The listing builds one solid part. Answer for the finished solid, in the listing's coordinates (mm). A direction names the side the tool comes from. Round coordinates to 2 decimals unless told otherwise and drop trailing zeros. Loops run counter-clockwise (first coordinate to the right, second up) from the corner with the lowest first, then second, coordinate; pieces in that order, holes last. Notation, with made-up numbers: (-35, 28) -> (-19, 28) arc R9 ccw to (-19, 35) -> close; hole circle Ø3 at (-25, 18). An arc over 180 degrees is marked (long way). Write each question's results on one line, items separated by ' | '. Start each with the question number.
(1) Flat-ended cylindrical pins translate along their axes: pin 1 (4 mm diameter, centred on y = -11.5, z = -11.5, fed in from +X); pin 2 (3 mm diameter, centred on x = 25.5, z = -13.5, fed in from +Y) (3 decimals); pin 3 (3.5 mm diameter, centred on x = 39.5, z = 0, fed in from +Y); pin 4 (2.5 mm diameter, centred on x = 5.5, y = -19.875, fed in from +Z). Find the tip coordinate at first contact, or state that the pin passes through.
(2) Straight lines are drawn through the part: probe 1 along Y at (x, z) = (5.5, -2.75) (3 decimals); probe 2 along Y at (x, z) = (39.5, 0.3); probe 3 along X at (y, z) = (-16.75, -3). For each, find the intervals that lie inside material, in ascending order.
(3) The part is cut by section B-B (z = 1). Determine the outline of the cut face in (x, y) (3 decimals).
(4) The part is cut by section D-D (y = -19.25). Determine the outline of the cut face in (x, z), plus the area to 3 significant figures.
(5) Determine the mould class of faces 4 (the face through (25, -11, 13.25)), 5 (the face through (25, -12.975, -14)), 6 (the face through (37, -11, -2)), 7 (the face through (24.73, -10.45, 15.78)) for opening direction Y: released by +Y, released by -Y, zero draft, split by the parting line, or undercut.
(6) The part is cut by section A-A (x = 5.5). Determine the outline of the cut face in (y, z) (3 decimals).
(7) The part is cut by section C-C (x = 25.47). Determine the outline of the cut face in (y, z) (3 decimals).
(8) For faces 1 (the face through (13, -9.8, -10.2)), 2 (the face through (14.24, -13.11, 10.24)), 3 (the face through (14, -11, -11.25)), determine the directions among +Z, -Z, +X, -X, +Y, -Y from which every point of the face is accessible in a straight line to the end or side of a thin tool.
Autodesk Inventor part; units mm, degrees
ref_plane "YZ Plane" through (0, 0, 0) normal (1, 0, 0) x (0, 1, 0)
ref_plane "XZ Plane" through (0, 0, 0) normal (0, 1, 0) x (-1, 0, 0)
ref_plane "XY Plane" through (0, 0, 0) normal (0, 0, 1) x (1, 0, 0)
sketch "Sketch1" plane through (0, 0, 0) normal (0, 0, 1) x (1, 0, 0)
  line L0 (0, 0) -> (32.875, 0)
  line L1 (37, 0) -> (37, -4.125)
  line L2 (37, -22.25) -> (0, -22.25)
  line L3 (0, -22.25) -> (0, -11.125)
  line L4 (0, -11.125) -> (37, -11.125) construction
  line L5 (0, -11.125) -> (0, 0)
  circle A0 centre (14.5, -11.125) radius 2
  circle A1 centre (5.5, -2.375) radius 1.5
  arc A2 (37, -4.125) -> (32.875, 0) centre (32.875, -4.125) ccw
  line L6 (32.875, 0) -> (37, 0)
  line L7 (37, -4.125) -> (37, -22.25)
  arc A3 (32.875, -22.25) -> (37, -18.125) centre (32.875, -18.125) ccw
  circle A4 centre (5.5, -19.875) radius 1.5
  circle A5 centre (25.47, -11.125) radius 2.7
  line L8 (23.5034, -9.275) -> (27.4366, -9.275)
  line L9 (27.4366, -12.975) -> (23.5034, -12.975)
  point P0 (36.5, -18.125)
  point P1 (36.9, -18.125)
  dimension "d6" = 4
  dimension "d8" = 3
  dimension "d11" = 5.5
  dimension "d12" = 22.25
  dimension "d13" = 8.75
  dimension "d16" = 14.5
  dimension "d17" = 14
  dimension "d18" = 37
  dimension "d19" = 3.7
  dimension "d28" = 5.4
  dimension "d29" = 11.53
extrude "Extrusion1" add sketch "Sketch1" along normal mid plane 18.5 contours L0 A2 L7 A3 L2 L3 L5
extrude "Extrusion2" add sketch "Sketch1" along normal mid plane 22.5 contours A0
extrude "Extrusion3" add sketch "Sketch1" along normal mid plane 20.5 contours A5 L9 L8 | L8 A5 | A5 L9
extrude "Extrusion4" add sketch "Sketch1" along normal mid plane 36.5 contours A5 L9 L8
sketch "Sketch2" plane through (0, -22.25, 9.25) normal (-1, 0, 0) x (0, 0, 1)
  point P0 (-9.25, 22.25)
sketch "Sketch3" plane through (0, 0, -18.25) normal (0, 0, -1) x (-1, 0, 0)
  circle A0 centre (-25.47, -11.125) radius 1
  arc A1 (-23.5034, -12.975) -> (-23.5034, -9.275) centre (-25.47, -11.125) ccw
  point P0 (0, 0)
  dimension "d30" = 2
extrude "Extrusion5" cut sketch "Sketch3" against normal blind 5
sketch "Sketch4" plane through (0, 0, 18.25) normal (0, 0, 1) x (1, 0, 0)
  circle A0 centre (25.47, -11.125) radius 1
  arc A1 (27.4366, -12.975) -> (27.4366, -9.275) centre (25.47, -11.125) ccw
  point P0 (0, 0)
  dimension "d33" = 2
extrude "Extrusion6" cut sketch "Sketch4" against normal blind 5
sketch "Sketch5" plane through (37, -18.125, 9.25) normal (1, 0, 0) x (0, 0, -1)
  line L0 (9.25, 18.125) -> (9.25, 0) construction
  line L1 (18.5, 0) -> (0, 0)
  line L2 (7.75, 9.625) -> (10.75, 9.625)
  line L3 (10.75, 9.625) -> (10.75, 4.625)
  line L4 (10.75, 4.625) -> (9.25, 4.625)
  line L5 (7.75, 4.625) -> (7.75, 9.625)
  line L6 (9.25, 4.625) -> (7.75, 4.625)
  dimension "d36" = 3
  dimension "d37" = 5
  dimension "d38" = 8.5
extrude "Extrusion7" add sketch "Sketch5" along normal blind 5
sketch "Sketch6" plane through (37, -13.5, 1.5) normal (0, 0, 1) x (1, 0, 0)
  circle A0 centre (2.5, 2.5) radius 1.5
  line L0 (5, 0) -> (5, 2.5) construction
  line L1 (5, 5) -> (5, 0) construction
  line L2 (5, 0) -> (5, 5) construction
  line L3 (5, 2.5) -> (0, 2.5) construction
  line L4 (5, 2.5) -> (5, 5) construction
  line L5 (5, 5) -> (5, 0) construction
  line L6 (0, 5) -> (5, 5) construction
  line L7 (2.5, 5) -> (2.5, 0) construction
  line L8 (0, 0) -> (5, 0)
  line L9 (0, 5) -> (0, 0) construction
  line L10 (0, 5) -> (0, 2.5) construction
  point P0 (-37, 13.5)
  point P1 (2.5, 2.5)
  dimension "d41" = 3
extrude "Extrusion8" cut sketch "Sketch6" against normal blind 5
ref_plane "Work Plane1" through (0, 0, 0) normal (0, 0, 1) x (1, 0, 0)
ref_plane "Work Plane2" through (0, -11.125, 9.25) normal (0, -1, 0) x (1, 0, 0)
properties part number "TT motor output"
Checked values:
1) pin 1: stops at x = 28.17 | pin 2: stops at y = -9.275 | pin 3: stops at y = -8.5 | pin 4: passes through
2) probe 1: y = -22.25 to -21.375, -18.375 to -3.875, -0.875 to 0 | probe 2: y = -13.5 to -12.5, -9.5 to -8.5 | probe 3: x = 0 to 37
3) outline: (0, -22.25) -> (32.875, -22.25) arc R4.125 ccw to (37, -18.125) -> (37, -13.5) -> (42, -13.5) -> (42, -8.5) -> (37, -8.5) -> (37, -4.125) arc R4.125 ccw to (32.875, 0) -> (0, 0) -> close; hole circle Ø3 at (5.5, -19.875); hole circle Ø3 at (5.5, -2.375); hole circle Ø3 at (39.5, -11)
4) outline: (0, -9.25) -> (4.14, -9.25) -> (4.14, 9.25) -> (0, 9.25) -> close; (6.86, -9.25) -> (36.84, -9.25) -> (36.84, 9.25) -> (6.86, 9.25) -> close | area: 631 mm2
5) face 4: undercut | face 5: released by -Y | face 6: zero draft | face 7: undercut
6) outline: (-22.25, -9.25) -> (-21.375, -9.25) -> (-21.375, 9.25) -> (-22.25, 9.25) -> close; (-18.375, -9.25) -> (-3.875, -9.25) -> (-3.875, 9.25) -> (-18.375, 9.25) -> close; (-0.875, -9.25) -> (0, -9.25) -> (0, 9.25) -> (-0.875, 9.25) -> close
7) outline: (-22.25, -9.25) -> (-13.825, -9.25) -> (-13.825, -10.25) -> (-12.975, -10.25) -> (-12.975, -18.25) -> (-12.125, -18.25) -> (-12.125, -13.25) -> (-10.125, -13.25) -> (-10.125, -18.25) -> (-9.275, -18.25) -> (-9.275, -10.25) -> (-8.425, -10.25) -> (-8.425, -9.25) -> (0, -9.25) -> (0, 9.25) -> (-8.425, 9.25) -> (-8.425, 10.25) -> (-9.275, 10.25) -> (-9.275, 18.25) -> (-10.125, 18.25) -> (-10.125, 13.25) -> (-12.125, 13.25) -> (-12.125, 18.25) -> (-12.975, 18.25) -> (-12.975, 10.25) -> (-13.825, 10.25) -> (-13.825, 9.25) -> (-22.25, 9.25) -> close
8) face 1: -Z | face 2: +Z | face 3: -Z, -X, +Y, -Y
